```python
from build123d import *

# Parameters (mm, degrees)
SKETCH_3_W          = 80
SKETCH_3_H          = 56
EXTRUDE_1_DEPTH     = 4.6
SKETCH_1_R          = 2.625
SKETCH_1_W          = 40.4
SKETCH_1_H          = 4.6
CUT_EXTRUDE_1_DEPTH = 4.6
SKETCH_5_R          = 4.85
EXTRUDE_2_DEPTH     = 25
SKETCH_6_R          = 2
EXTRUDE_3_DEPTH     = 8
FILLET_2_R          = 4


with BuildPart() as part:
    # 草图3 → 凸台-拉伸1 (new body)
    with BuildSketch(Plane(origin=(0, 0, 0), x_dir=(1, 0, 0), z_dir=(0, 1, 0))):
        Rectangle(SKETCH_3_W, SKETCH_3_H)
    extrude(amount=EXTRUDE_1_DEPTH)

    # 草图1 → 切除-拉伸1 (cut)
    with BuildSketch(Plane(origin=(0, 0, 0), x_dir=(1, 0, 0), z_dir=(0, 1, 0))):
        with Locations(Location((-31.75, 20.6375, 0), (0, 0, 90))):
            Circle(SKETCH_1_R)
        with Locations(Location((31.75, 20.6375, 0), (0, 0, 90))):
            Circle(SKETCH_1_R)
        with Locations(Location((31.75, -20.6375, 0), (0, 0, 90))):
            Circle(SKETCH_1_R)
        with Locations(Location((-31.75, -20.6375, 0), (0, 0, 90))):
            Circle(SKETCH_1_R)
        with Locations(Location((-22.225, 20.6375, 0), (0, 0, 90))):
            Circle(SKETCH_1_R)
        with Locations(Location((-22.225, -20.6375, 0), (0, 0, 90))):
            Circle(SKETCH_1_R)
        with Locations((0, -10.4375)):
            Rectangle(SKETCH_1_W, SKETCH_1_H)
        with Locations((0, 10.4375)):
            Rectangle(SKETCH_1_W, SKETCH_1_H)
    extrude(amount=CUT_EXTRUDE_1_DEPTH, mode=Mode.SUBTRACT)

    # 草图5 → 凸台-拉伸2 (add)
    with BuildSketch(Plane.XZ):
        with Locations(Location((31.75, 20.6375, 0), (0, 0, 270))):
            Circle(SKETCH_5_R)
    extrude(amount=EXTRUDE_2_DEPTH)

    # 草图6 → 凸台-拉伸3 (add)
    with BuildSketch(Plane.XZ.offset(25)):
        with Locations(Location((31.75, 20.6375, 0), (0, 0, 270))):
            Circle(SKETCH_6_R)
    extrude(amount=EXTRUDE_3_DEPTH)

    # 圆角2
    fillet_2_edges = [part.edges().sort_by_distance(p)[0] for p in [
        (40, 2.3, 28),
        (-40, 2.3, 28),
        (-40, 2.3, -28),
        (40, 2.3, -28),
    ]]
    fillet(fillet_2_edges, radius=FILLET_2_R)


solid = part.part
```
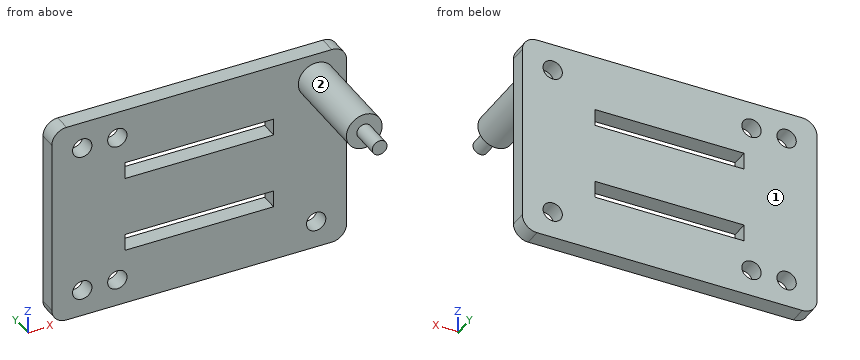
Geometry check sheet. Reference: the model listing, model coordinates, mm. Face numbers are marked on the shaded views. A direction names the side the tool comes from. Round coordinates to 2 decimals unless told otherwise and drop trailing zeros. Write each loop counter-clockwise with the first axis right and the second up, starting at its lowest first coordinate (ties: lowest second). Pieces come first, ordered by that corner, then holes. Notation, with made-up numbers: (25, 48.5) -> (57, 48.5) arc R29 cw to (57, 80.5) -> close; hole circle Ø10 at (3.5, 20.5). An arc over 180 degrees is marked (long way). Put each result on its own line as item: value.
1) Cross-section at A-A, the plane x = -9. Enter the section's corners in (y, z), plus the area to 3 significant figures.
Recorded:
outline: (0, -28) -> (4.6, -28) -> (4.6, -12.74) -> (0, -12.74) -> close; (0, -8.14) -> (4.6, -8.14) -> (4.6, 8.14) -> (0, 8.14) -> close; (0, 12.74) -> (4.6, 12.74) -> (4.6, 28) -> (0, 28) -> close
area: 215 mm2
2) Access from +Z, -Z, +X, -X, +Y, -Y to the whole of each face (thin tool, end or side, straight path). Record for the marked faces 1 and 2.
Recorded:
face 1: +Z, -Z, +X, -X, +Y
face 2: -Y
3) Thickness scan on probe 1 along Z at (x, y) = (-31.75, 1.1); probe 2 along Y at (x, z) = (33.5, 1.5); probe 3 along X at (y, z) = (-22, 23). Record the ranges inside material, lowest first. Write a range as from..to.
Recorded:
probe 1: z = -28..-23.26, -18.01..18.01, 23.26..28
probe 2: y = 0..4.6
probe 3: x = 27.51..35.99
4) Cross-section at C-C, the plane z = 10. Enter the section's corners in (x, y).
Recorded:
outline: (-40, 0) -> (-20.2, 0) -> (-20.2, 4.6) -> (-40, 4.6) -> close; (20.2, 0) -> (40, 0) -> (40, 4.6) -> (20.2, 4.6) -> close
5) Cross-section at B-B, the plane x = 31.75. Enter the section's corners in (y, z), plus the area to 3 significant figures.
Recorded:
outline: (-33, 18.64) -> (-25, 18.64) -> (-25, 15.79) -> (0, 15.79) -> (0, -18.01) -> (4.6, -18.01) -> (4.6, 18.01) -> (0, 18.01) -> (0, 23.26) -> (4.6, 23.26) -> (4.6, 28) -> (0, 28) -> (0, 25.49) -> (-25, 25.49) -> (-25, 22.64) -> (-33, 22.64) -> close; (0, -28) -> (4.6, -28) -> (4.6, -23.26) -> (0, -23.26) -> close
area: 484 mm2
6) Depth check by flat-ended pin: P1, Ø1, axis at y = -9.5, z = 17, coming from the +X side; P2, Ø4, axis at x = -28, z = -6, coming from the -Y side; P3, Ø4, axis at x = -31.75, z = 20.64, coming from the -Y side; P4, Ø1.6, axis at x = 32.5, z = 21, coming from the +Y side. Enter the tip coordinate at first touch or a pass-through.
Recorded:
P1: stops at x = 35.45
P2: stops at y = 0
P3: passes through
P4: stops at y = 0
7) Cross-section at D-D, the plane x = -31.75. Enter the section's corners in (y, z), plus the area to 3 significant figures.
Recorded:
outline: (0, -28) -> (4.6, -28) -> (4.6, -23.26) -> (0, -23.26) -> close; (0, -18.01) -> (4.6, -18.01) -> (4.6, 18.01) -> (0, 18.01) -> close; (0, 23.26) -> (4.6, 23.26) -> (4.6, 28) -> (0, 28) -> close
area: 209 mm2
